CAD build for the part. Positions are in the model's coordinates, mm. A direction names the side the tool comes from. Give positions to 0.01 mm unless a question says otherwise; leave off trailing zeros. Loops run counter-clockwise (first coordinate to the right, second up) from the corner with the lowest first, then second, coordinate; pieces in that order, holes last. Notation, with made-up numbers: M 6.5,86.25 L 35.5,86.25 A14 ccw 35.5,100.25 Z; hole C 60,71.5 d11. An arc over 180 degrees is marked long. Answer as CSV lines item,"result".
```python
from build123d import *
from build123d.topology import SkipClean

# Parameters (mm, degrees)
EXTRUDE_1_DEPTH = 0.5
EXTRUDE_2_DEPTH = 6.4
EXTRUDE_3_DEPTH = 0.5
EXTRUDE_START   = -7.4
EXTRUDE_6_DEPTH = 7.4
EXTRUDE_7_DEPTH = 6.4
EXTRUDE_8_DEPTH = 0.5


with BuildPart() as part:
    # 草图1 → 凸台-拉伸1 (new body)
    with BuildSketch(Plane(origin=(0, 0, 0), x_dir=(1, 0, 0), z_dir=(0, 1, 0))):
        with BuildLine():
            Line((10.958141679, 0.95871317), (9.961946981, 0.871557427))
            ThreePointArc((9.961946981, 0.871557427), (-10, 0), (9.961946981, -0.871557427))
            Line((9.961946981, -0.871557427), (10.958141679, -0.95871317))
            ThreePointArc((10.958141679, -0.95871317), (5.079234746, -9.757119165), (-5.5, -9.526279442))
            Line((-5.5, -9.526279442), (-7, -12.124355653))
            ThreePointArc((-7, -12.124355653), (-8.522660006, -11.106946764), (-9.899494937, -9.899494937))
            Line((-9.899494937, -9.899494937), (-7.778174593, -7.778174593))
            ThreePointArc((-7.778174593, -7.778174593), (-9.969385657, -4.648800879), (-10.958141679, -0.95871317))
            Line((-10.958141679, -0.95871317), (-12.950531075, -1.133024656))
            ThreePointArc((-12.950531075, -1.133024656), (-13, 0), (-12.950531075, 1.133024656))
            Line((-12.950531075, 1.133024656), (-10.958141679, 0.95871317))
            ThreePointArc((-10.958141679, 0.95871317), (-9.969385657, 4.648800879), (-7.778174593, 7.778174593))
            Line((-7.778174593, 7.778174593), (-9.899494937, 9.899494937))
            ThreePointArc((-9.899494937, 9.899494937), (-8.522660006, 11.106946764), (-7, 12.124355653))
            Line((-7, 12.124355653), (-5.5, 9.526279442))
            ThreePointArc((-5.5, 9.526279442), (5.079234746, 9.757119165), (10.958141679, 0.95871317))
        make_face()
    extrude(amount=EXTRUDE_1_DEPTH)

    # 草图10 → 凸台-拉伸2 (add)
    with BuildSketch(Plane(origin=(0, 0.5, 0), x_dir=(1, 0, 0), z_dir=(0, 1, 0))):
        with BuildLine():
            Line((9.961946981, -0.871557427), (10.958141679, -0.95871317))
            ThreePointArc((10.958141679, -0.95871317), (9.757119165, -5.079234746), (7.070663707, -8.426488874))
            Line((7.070663707, -8.426488874), (6.427876097, -7.660444431))
            ThreePointArc((6.427876097, -7.660444431), (8.870108332, -4.617486132), (9.961946981, -0.871557427))
        make_face()
        with BuildLine():
            Line((9.961946981, 0.871557427), (10.958141679, 0.95871317))
            ThreePointArc((10.958141679, 0.95871317), (9.744466641, 5.103466458), (7.028695203, 8.46152727))
            Line((7.028695203, 8.46152727), (6.389722912, 7.692297518))
            ThreePointArc((6.389722912, 7.692297518), (8.858606037, 4.639514962), (9.961946981, 0.871557427))
        make_face()
        with BuildLine():
            Line((6.314487726, -9.007066379), (5.704869745, -8.213066491))
            ThreePointArc((5.704869745, -8.213066491), (-9.999967824, -0.025367673), (5.663127179, 8.241904547))
            Line((5.663127179, 8.241904547), (6.268753512, 9.038956212))
            ThreePointArc((6.268753512, 9.038956212), (-10.999964675, -0.027877319), (6.314487726, -9.007066379))
        make_face()
    extrude(amount=EXTRUDE_2_DEPTH)

    # 草图11 → 凸台-拉伸3 (add)
    with SkipClean():  # the faces are left unmerged after this step: merging them gives an invalid solid
        with BuildSketch(Plane(origin=(0, 6.9, 0), x_dir=(1, 0, 0), z_dir=(0, 1, 0))):
            with BuildLine():
                Line((9.961946981, 0.871557427), (10.958141679, 0.95871317))
                ThreePointArc((10.958141679, 0.95871317), (-11, 0), (10.958141679, -0.95871317))
                Line((10.958141679, -0.95871317), (9.961946981, -0.871557427))
                ThreePointArc((9.961946981, -0.871557427), (-10, 0), (9.961946981, 0.871557427))
            make_face()
        extrude(amount=EXTRUDE_3_DEPTH)

    # 草图14 → 凸台-拉伸6 (add)
    with SkipClean():  # the faces are left unmerged after this step: merging them gives an invalid solid
        with BuildSketch(Plane(origin=(0, 7.4, 0), x_dir=(1, 0, 0), z_dir=(0, 1, 0)).offset(EXTRUDE_START)):
            with BuildLine():
                Line((9.961946981, 0.871557427), (10.958141679, 0.95871317))
                ThreePointArc((10.958141679, 0.95871317), (11, 0), (10.958141679, -0.95871317))
                Line((10.958141679, -0.95871317), (9.961946981, -0.871557427))
                ThreePointArc((9.961946981, -0.871557427), (10, 0), (9.961946981, 0.871557427))
            make_face()
        extrude(amount=EXTRUDE_6_DEPTH)

    # 草图12 → 凸台-拉伸7 (add)
    with SkipClean():  # the faces are left unmerged after this step: merging them gives an invalid solid
        with BuildSketch(Plane(origin=(0, 0.5, 0), x_dir=(1, 0, 0), z_dir=(0, 1, 0))):
            with BuildLine():
                Line((-7.778174593, -7.778174593), (-8.485281374, -8.485281374))
                ThreePointArc((-8.485281374, -8.485281374), (-7.305137148, -9.520240083), (-6, -10.392304845))
                Line((-6, -10.392304845), (-5.5, -9.526279442))
                ThreePointArc((-5.5, -9.526279442), (-6.696375719, -8.726886743), (-7.778174593, -7.778174593))
            make_face()
            with BuildLine():
                Line((-9.899494937, -9.899494937), (-9.333809512, -9.333809512))
                ThreePointArc((-9.333809512, -9.333809512), (-8.035650863, -10.472264092), (-6.6, -11.43153533))
                Line((-6.6, -11.43153533), (-7, -12.124355653))
                ThreePointArc((-7, -12.124355653), (-8.522660006, -11.106946764), (-9.899494937, -9.899494937))
            make_face()
            with BuildLine():
                Line((-9.899494937, 9.899494937), (-9.333809512, 9.333809512))
                ThreePointArc((-9.333809512, 9.333809512), (-8.035650863, 10.472264092), (-6.6, 11.43153533))
                Line((-6.6, 11.43153533), (-7, 12.124355653))
                ThreePointArc((-7, 12.124355653), (-8.522660006, 11.106946764), (-9.899494937, 9.899494937))
            make_face()
            with BuildLine():
                Line((-5.5, 9.526279442), (-6, 10.392304845))
                ThreePointArc((-6, 10.392304845), (-7.305137148, 9.520240083), (-8.485281374, 8.485281374))
                Line((-8.485281374, 8.485281374), (-7.778174593, 7.778174593))
                ThreePointArc((-7.778174593, 7.778174593), (-6.696375719, 8.726886743), (-5.5, 9.526279442))
            make_face()
            with BuildLine():
                Line((-12.950531075, 1.133024656), (-11.954336377, 1.045868913))
                ThreePointArc((-11.954336377, 1.045868913), (-12, 0), (-11.954336377, -1.045868913))
                Line((-11.954336377, -1.045868913), (-12.950531075, -1.133024656))
                ThreePointArc((-12.950531075, -1.133024656), (-13, 0), (-12.950531075, 1.133024656))
            make_face()
        extrude(amount=EXTRUDE_7_DEPTH)

    # 草图15 → 凸台-拉伸8 (add)
    with SkipClean():  # the faces are left unmerged after this step: merging them gives an invalid solid
        with BuildSketch(Plane(origin=(0, 6.9, 0), x_dir=(1, 0, 0), z_dir=(0, 1, 0))):
            with BuildLine():
                Line((-12.950531075, 1.133024656), (-10.958141679, 0.95871317))
                ThreePointArc((-10.958141679, 0.95871317), (-11, 0), (-10.958141679, -0.95871317))
                Line((-10.958141679, -0.95871317), (-12.950531075, -1.133024656))
                ThreePointArc((-12.950531075, -1.133024656), (-13, 0), (-12.950531075, 1.133024656))
            make_face()
            with BuildLine():
                Line((-9.899494937, -9.899494937), (-7.778174593, -7.778174593))
                ThreePointArc((-7.778174593, -7.778174593), (-6.696375719, -8.726886743), (-5.5, -9.526279442))
                Line((-5.5, -9.526279442), (-7, -12.124355653))
                ThreePointArc((-7, -12.124355653), (-8.522660006, -11.106946764), (-9.899494937, -9.899494937))
            make_face()
            with BuildLine():
                Line((-9.899494937, 9.899494937), (-7.778174593, 7.778174593))
                ThreePointArc((-7.778174593, 7.778174593), (-6.696375719, 8.726886743), (-5.5, 9.526279442))
                Line((-5.5, 9.526279442), (-7, 12.124355653))
                ThreePointArc((-7, 12.124355653), (-8.522660006, 11.106946764), (-9.899494937, 9.899494937))
            make_face()
        extrude(amount=EXTRUDE_8_DEPTH)


solid = part.part
```
Q1. Cut at D-D (z = 7). Write the cut outline in (x, y).
Solution:
outline,"M -8.49,0 L -7.14,0 L -7.14,7.4 L -8.49,7.4 Z; M 7.14,0 L 8.49,0 L 8.49,7.4 L 7.14,7.4 Z"
Q2. Mould opens along Y. For faces 1 (the flat face through (-8, 4, 8)), 2 (the flat face through (6.4, 0.5, -8.4)), 3 (the flat face through (-9, 0, -5)) say: released by +Y, released by -Y, zero draft, split by the parting line, or undercut.
Solution:
face 1,"zero draft"
face 2,"undercut"
face 3,"released by -Y"
Q3. Wall check: line 1 (Z direction, x = 0, y = 4); line 2 (Y direction, x = -8.5, z = -9.25); line 3 (X direction, y = 0.2, z = 0). Give the ranges that are in metal, low to high. Write a range as [from, to].
Solution:
line 1,"z = [-11, -10], [10, 11]"
line 2,"y = [0, 0.5], [6.9, 7.4]"
line 3,"x = [-13, -10], [10, 11]"
Q4. Pin check, flat tips, straight feed: P1, Ø2, axis at y = 4, z = -4.5, coming from the -X side; P2, Ø1.5, axis at y = 4.5, z = 5, coming from the -X side. Stop position of each tip, or through.
Solution:
P1,"stops at x = -10.43"
P2,"stops at x = -10.15"
Q5. Cut at A-A (z = 0). Write the cut outline in (x, y), and give its area (3 significant figures).
Solution:
outline,"M -13,0 L -10,0 L -10,7.4 L -13,7.4 Z; M 10,0 L 11,0 L 11,7.4 L 10,7.4 Z; hole M -12,0.5 L -11,0.5 L -11,6.9 L -12,6.9 Z"
area,"23.2 mm²"
Q6. Cut at B-B (x = 0). Write the cut outline in (y, z), and give its area (3 significant figures).
Solution:
outline,"M 0,-11 L 7.4,-11 L 7.4,-10 L 0,-10 Z; M 0,10 L 7.4,10 L 7.4,11 L 0,11 Z"
area,"14.8 mm²"
Q7. Cut at C-C (y = 6). Write the cut outline in (x, z), and give its area (3 significant figures).
Solution:
outline,"M -12.95,-1.13 L -11.95,-1.05 A12 cw -11.95,1.05 L -12.95,1.13 A13 ccw Z; M -9.9,-9.9 A14 ccw -7,-12.12 L -6.6,-11.43 A13.2 cw -9.33,-9.33 Z; M -9.9,9.9 L -9.33,9.33 A13.2 cw -6.6,11.43 L -7,12.12 A14 ccw Z; M -8.49,-8.49 A12 ccw -6,-10.39 L -5.5,-9.53 A11 ccw 6.27,-9.04 L 5.66,-8.24 A10 cw long 5.7,8.21 L 6.31,9.01 A11 ccw -5.5,9.53 L -6,10.39 A12 ccw -8.49,8.49 L -7.78,7.78 A11 ccw -7.78,-7.78 Z; M 6.39,-7.69 L 7.03,-8.46 A11 ccw 7.07,8.43 L 6.43,7.66 A10 cw Z"
area,"78.0 mm²"
Q8. Which spindle directions (+Z, -Z, +X, -X, +Y, -Y) get a long thin tool onto all of the face, cutting with end or side? Do faces 4 (the flat face through (-8, 6.9, 10)), 5 (the cylindrical face through (-8.502, 3.648, -11.123)), 6 (the flat face through (-12.19, 3.648, -1.066)). Say none if no direction does.
Solution:
face 4,"none"
face 5,"-Z, -X, +Y, -Y"
face 6,"-Z, +Y, -Y"
